Source: CAD feature listing. Evaluate the final solid. Frame: model axes, mm. Face numbers are marked on the shaded views. A direction names the side the tool comes from. Give positions to 0.01 mm unless a question says otherwise; leave off trailing zeros. Order: outer loops, then holes, each group sorted by start corner. A loop starts at its lowest first (then second) coordinate and runs counter-clockwise, first axis right, second up.
```python
from build123d import *

# Parameters (mm, degrees)
SKETCH_W        = 65
SKETCH_H        = 25
PAD_DEPTH       = 20
SKETCH001_W     = 65
SKETCH001_H     = 3.5
POCKET_DEPTH    = 7.5
SKETCH002_W     = 40
SKETCH002_H     = 7
POCKET001_DEPTH = 10
SKETCH003_W     = 35
SKETCH003_H     = 12.5
POCKET002_DEPTH = 14
CHAMFER_SIZE    = 4
CHAMFER001_SIZE = 4
FILLET_R        = 3.9
FILLET001_R     = 2
FILLET002_R     = 1.5
FILLET003_R     = 3
FILLET004_R     = 6
FILLET005_R     = 1


with BuildPart() as part:
    # Sketch → Pad (new body)
    with BuildSketch(Plane.XY):
        with Locations((32.5, 12.5)):
            Rectangle(SKETCH_W, SKETCH_H)
    extrude(amount=PAD_DEPTH)

    # Sketch001 → Pocket (cut)
    with BuildSketch(Plane.XY.offset(20)):
        with Locations((32.5, 12.5)):
            Rectangle(SKETCH001_W, SKETCH001_H)
    extrude(amount=-POCKET_DEPTH, mode=Mode.SUBTRACT)

    # Sketch002 → Pocket001 (cut)
    with BuildSketch(Plane.XY.offset(20)):
        with Locations((45, 12.5)):
            Rectangle(SKETCH002_W, SKETCH002_H)
    extrude(amount=-POCKET001_DEPTH, mode=Mode.SUBTRACT)

    # Sketch003 → Pocket002 (cut)
    with BuildSketch(Plane.XY.offset(20)):
        with Locations((47.5, 12.5)):
            Rectangle(SKETCH003_W, SKETCH003_H)
    extrude(amount=-POCKET002_DEPTH, mode=Mode.SUBTRACT)

    # Chamfer
    chamfer_edges = [part.edges().sort_by_distance(p)[0] for p in [
        (65, 25, 10),
        (65, 0, 10),
    ]]
    chamfer(chamfer_edges, length=CHAMFER_SIZE)

    # Chamfer001
    chamfer001_edges = [part.edges().sort_by_distance(p)[0] for p in [
        (30.5, 0, 0),
        (30.5, 25, 0),
    ]]
    chamfer(chamfer001_edges, length=CHAMFER001_SIZE)

    # Fillet
    fillet_edges = [part.edges().sort_by_distance(p)[0] for p in [
        (61, 0, 12),
        (30.5, 0, 4),
        (30.5, 0, 20),
        (0, 0, 12),
        (61, 25, 12),
        (30.5, 25, 4),
        (30.5, 25, 20),
        (0, 25, 12),
    ]]
    fillet(fillet_edges, radius=FILLET_R)

    # Fillet001
    fillet001_edges = [part.edges().sort_by_distance(p)[0] for p in [
        (0, 7.325, 20),
        (0, 17.675, 20),
    ]]
    fillet(fillet001_edges, radius=FILLET001_R)

    # Fillet002
    fillet002_edges = [part.edges().sort_by_distance(p)[0] for p in [
        (12.5, 14.25, 12.5),
        (12.5, 10.75, 12.5),
    ]]
    fillet(fillet002_edges, radius=FILLET002_R)

    # Fillet003
    fillet003_edges = [part.edges().sort_by_distance(p)[0] for p in [
        (27.5, 9, 10),
        (27.5, 16, 10),
    ]]
    fillet(fillet003_edges, radius=FILLET003_R)

    # Fillet004
    fillet004_edges = [part.edges().sort_by_distance(p)[0] for p in [
        (47.5, 18.75, 6),
        (47.5, 6.25, 6),
    ]]
    fillet(fillet004_edges, radius=FILLET004_R)

    # Fillet005
    fillet005_edges = [part.edges().sort_by_distance(p)[0] for p in [
        (13.5, 14.25, 20),
        (13.5, 10.75, 20),
        (27.5, 16, 20),
        (27.5, 9, 20),
        (47.5, 18.75, 20),
        (47.5, 6.25, 20),
    ]]
    fillet(fillet005_edges, radius=FILLET005_R)


solid = part.part
```
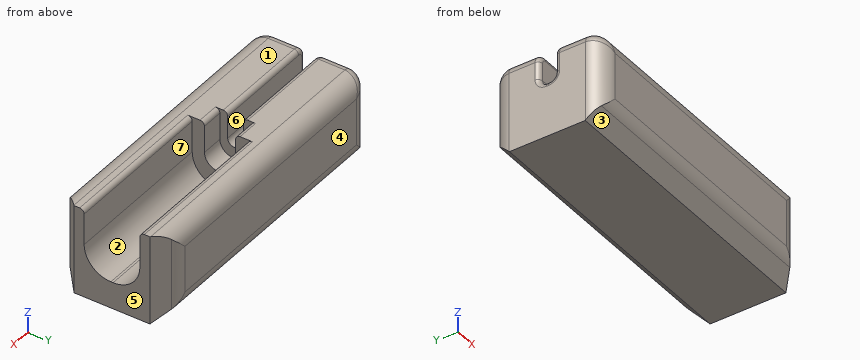
1) Pin query (flat end, axial travel): pin 1 (4 mm diameter, centred on x = 40.5, z = 5, fed in from +Y); pin 2 (10 mm diameter, centred on y = 13, z = 17.5, fed in from +X); pin 3 (0.5 mm diameter, centred on x = 28, y = 12.5, fed in from +Z). Return the tip coordinate at first contact, or that it passes through.
Report:
pin 1: stops at y = 25
pin 2: stops at x = 30
pin 3: stops at z = 10
2) Section query B-B, the plane x = 11. Return the cut outline in (y, z).
Report:
outline: (0, 5.62) arc R3.9 ccw to (1.14, 2.86) - (4, 0) - (21, 0) - (23.86, 2.86) arc R3.9 ccw to (25, 5.62) - (25, 16.1) arc R3.9 ccw to (21.1, 20) - (15.25, 20) arc R1 ccw to (14.25, 19) - (14.25, 14) arc R1.5 cw to (12.75, 12.5) - (12.25, 12.5) arc R1.5 cw to (10.75, 14) - (10.75, 19) arc R1 ccw to (9.75, 20) - (3.9, 20) arc R3.9 ccw to (0, 16.1) - close
3) Section query C-C, the plane z = 3.75. Return the cut outline in (x, y), and give its area (3 significant figures).
Report:
outline: (0, 3.9) arc R3.9 ccw to (2.03, 0.48) - (61.25, 0.48) arc R3.9 ccw to (62.14, 1.14) - (65, 4) - (65, 21) - (62.14, 23.86) arc R3.9 ccw to (61.25, 24.52) - (2.03, 24.52) arc R3.9 ccw to (0, 21.1) - close
area: 1,550 mm2
4) Reachability of the marked faces 5, 6 and 7 from +Z, -Z, +X, -X, +Y, -Y: full face, straight path, thin tool, end or side. Return the list, or none.
Report:
face 5: +Z, -Z, +X, +Y, -Y
face 6: +Z, +X, -X
face 7: +Z, +X
5) Section query A-A, the plane z = 15.5. Return the cut outline in (x, y), and give its area (3 significant figures).
Report:
outline: (0, 3.9) arc R3.9 ccw to (3.9, 0) - (59.38, 0) arc R3.9 ccw to (62.14, 1.14) - (65, 4) - (65, 6.25) - (30, 6.25) - (30, 9) - (25, 9) - (25, 10.75) - (1, 10.75) arc R1 ccw to (0, 9.75) - close; (0, 15.25) arc R1 ccw to (1, 14.25) - (25, 14.25) - (25, 16) - (30, 16) - (30, 18.75) - (65, 18.75) - (65, 21) - (62.14, 23.86) arc R3.9 ccw to (59.38, 25) - (3.9, 25) arc R3.9 ccw to (0, 21.1) - close
area: 1,040 mm2
6) Material intervals for L1, parallel to Y at x = 31, z = 12.75; L2, parallel to Y at x = 23, z = 14.75; L3, parallel to Z at x = 31.5, y = 10.5, sorted ascending.
Report:
L1: y = 0 to 6.25, 18.75 to 25
L2: y = 0 to 10.75, 14.25 to 25
L3: z = 0 to 6.26
7) Section query D-D, the plane x = 49. Return the cut outline in (y, z).
Report:
outline: (0, 5.62) arc R3.9 ccw to (1.14, 2.86) - (4, 0) - (21, 0) - (23.86, 2.86) arc R3.9 ccw to (25, 5.62) - (25, 16.1) arc R3.9 ccw to (21.1, 20) - (19.75, 20) arc R1 ccw to (18.75, 19) - (18.75, 12) arc R6 cw to (12.75, 6) - (12.25, 6) arc R6 cw to (6.25, 12) - (6.25, 19) arc R1 ccw to (5.25, 20) - (3.9, 20) arc R3.9 ccw to (0, 16.1) - close
8) Draft query along Y for the marked faces 1, 2, 3 and 4. Return one class per face: +Y half, -Y half, draft (parallel to the pull), parting line (faces both ways), or undercut.
Report:
face 1: draft
face 2: undercut
face 3: -Y half
face 4: +Y half
